```python
from build123d import *

# Parameters (mm, degrees)
SKETCH_1_R          = 1.1
SKETCH_1_R_2        = 1.35
EXTRUDE_1_DEPTH     = 3
SKETCH_2_R          = 1.6
CUT_EXTRUDE_1_DEPTH = 177.943493805
CUT_EXTRUDE_2_DEPTH = 177.943493805
FILLET_1_R          = 3
FILLET_2_R          = 1
FILLET_3_R          = 20


with BuildPart() as part:
    # 草图1 → 凸台-拉伸1 (new body)
    with BuildSketch(Plane(origin=(0, 0, 0), x_dir=(1, 0, 0), z_dir=(0, 1, 0))):
        Polygon((20, 120), (20, 80), (110, 80), (110, 120), (130, 120), (130, 0), (0, 0), (0, 120), align=None)
        with Locations(Location((10, 115, 0), (0, 0, 270))):
            Circle(SKETCH_1_R, mode=Mode.SUBTRACT)
        with Locations(Location((120, 115, 0), (0, 0, 90))):
            Circle(SKETCH_1_R, mode=Mode.SUBTRACT)
        with Locations(Location((10, 100, 0), (0, 0, 270))):
            Circle(SKETCH_1_R, mode=Mode.SUBTRACT)
        with Locations(Location((120, 100, 0), (0, 0, 90))):
            Circle(SKETCH_1_R, mode=Mode.SUBTRACT)
        with Locations(Location((10, 85, 0), (0, 0, 270))):
            Circle(SKETCH_1_R, mode=Mode.SUBTRACT)
        with Locations(Location((120, 85, 0), (0, 0, 90))):
            Circle(SKETCH_1_R, mode=Mode.SUBTRACT)
        with Locations(Location((10, 70, 0), (0, 0, 270))):
            Circle(SKETCH_1_R, mode=Mode.SUBTRACT)
        with Locations(Location((120, 70, 0), (0, 0, 90))):
            Circle(SKETCH_1_R, mode=Mode.SUBTRACT)
        with Locations(Location((10, 55, 0), (0, 0, 270))):
            Circle(SKETCH_1_R, mode=Mode.SUBTRACT)
        with Locations(Location((120, 55, 0), (0, 0, 90))):
            Circle(SKETCH_1_R, mode=Mode.SUBTRACT)
        with Locations(Location((10, 40, 0), (0, 0, 270))):
            Circle(SKETCH_1_R, mode=Mode.SUBTRACT)
        with Locations(Location((120, 40, 0), (0, 0, 90))):
            Circle(SKETCH_1_R, mode=Mode.SUBTRACT)
        with Locations(Location((50, 57.5, 0), (0, 0, 270))):
            Circle(SKETCH_1_R_2, mode=Mode.SUBTRACT)
        with Locations(Location((50, 43.5, 0), (0, 0, 270))):
            Circle(SKETCH_1_R_2, mode=Mode.SUBTRACT)
        with Locations(Location((80, 43.5, 0), (0, 0, 90))):
            Circle(SKETCH_1_R_2, mode=Mode.SUBTRACT)
        with Locations(Location((80, 57.5, 0), (0, 0, 90))):
            Circle(SKETCH_1_R_2, mode=Mode.SUBTRACT)
    extrude(amount=EXTRUDE_1_DEPTH)

    # 草图2 → 切除-拉伸1 (cut, through all)
    with BuildSketch(Plane.XZ):
        with Locations(Location((24, -7.85, 0), (0, 0, 270))):
            Circle(SKETCH_2_R)
        with Locations(Location((35, -7.85, 0), (0, 0, 90))):
            Circle(SKETCH_2_R)
        with Locations(Location((35, -67.85, 0), (0, 0, 270))):
            Circle(SKETCH_2_R)
        with Locations(Location((24, -67.85, 0), (0, 0, 90))):
            Circle(SKETCH_2_R)
        with Locations(Location((95, -67.85, 0), (0, 0, 90))):
            Circle(SKETCH_2_R)
        with Locations(Location((106, -67.85, 0), (0, 0, 270))):
            Circle(SKETCH_2_R)
        with Locations(Location((95, -7.85, 0), (0, 0, 270))):
            Circle(SKETCH_2_R)
        with Locations(Location((106, -7.85, 0), (0, 0, 90))):
            Circle(SKETCH_2_R)
        Polygon((37.954915028, -15.35), (29.5, -32.259830056), (21.045084972, -15.35), align=None)
        Polygon((19.5, -23.440169944), (26.704915028, -37.85), (19.5, -52.259830056), align=None)
        Polygon((29.5, -43.440169944), (21.045084972, -60.35), (37.954915028, -60.35), align=None)
        Polygon((90.5, -23.440169944), (97.704915028, -37.85), (90.5, -52.259830056), align=None)
        Polygon((39.5, -23.440169944), (39.5, -52.259830056), (32.295084972, -37.85), align=None)
        Polygon((100.5, -43.440169944), (92.045084972, -60.35), (108.954915028, -60.35), align=None)
        Polygon((110.5, -23.440169944), (103.295084972, -37.85), (110.5, -52.259830056), align=None)
        Polygon((92.045084972, -15.35), (108.954915028, -15.35), (100.5, -32.259830056), align=None)
        Polygon((54.545084972, -13.5), (75.454915028, -13.5), (65, -34.409830056), align=None)
        Polygon((53, -21.590169944), (62.204915028, -40), (53, -58.409830056), align=None)
        Polygon((65, -45.590169944), (76.079915028, -67.75), (53.920084972, -67.75), align=None)
        Polygon((77, -21.590169944), (77, -58.409830056), (67.795084972, -40), align=None)
    extrude(amount=-CUT_EXTRUDE_1_DEPTH, mode=Mode.SUBTRACT)

    # 草图3 → 切除-拉伸2 (cut, through all)
    with BuildSketch(Plane(origin=(0, 3, 0), x_dir=(1, 0, 0), z_dir=(0, 1, 0))):
        Polygon((17, 0), (0, 40), (0, 0), align=None)
        Polygon((113, 0), (130, 40), (130, 0), align=None)
    extrude(amount=-CUT_EXTRUDE_2_DEPTH, mode=Mode.SUBTRACT)

    # 圆角1
    fillet_1_edges = [part.edges().sort_by_distance(p)[0] for p in [
        (0, 1.5, -120),
        (20, 1.5, -120),
        (110, 1.5, -120),
        (130, 1.5, -120),
        (17, 1.5, 0),
        (0, 1.5, -40),
        (113, 1.5, 0),
        (130, 1.5, -40),
    ]]
    fillet(fillet_1_edges, radius=FILLET_1_R)

    # 圆角2
    fillet_2_edges = [part.edges().sort_by_distance(p)[0] for p in [
        (90.5, 1.5, -52.259830056),
        (90.5, 1.5, -23.440169944),
        (97.704915028, 1.5, -37.85),
        (19.5, 1.5, -52.259830056),
        (19.5, 1.5, -23.440169944),
        (26.704915028, 1.5, -37.85),
        (21.045084972, 1.5, -15.35),
        (37.954915028, 1.5, -15.35),
        (29.5, 1.5, -32.259830056),
        (39.5, 1.5, -52.259830056),
        (32.295084972, 1.5, -37.85),
        (39.5, 1.5, -23.440169944),
        (53.920084972, 1.5, -67.75),
        (65, 1.5, -45.590169944),
        (76.079915028, 1.5, -67.75),
        (100.5, 1.5, -32.259830056),
        (92.045084972, 1.5, -15.35),
        (108.954915028, 1.5, -15.35),
        (100.5, 1.5, -43.440169944),
        (108.954915028, 1.5, -60.35),
        (92.045084972, 1.5, -60.35),
        (110.5, 1.5, -23.440169944),
        (110.5, 1.5, -52.259830056),
        (103.295084972, 1.5, -37.85),
        (37.954915028, 1.5, -60.35),
        (21.045084972, 1.5, -60.35),
        (29.5, 1.5, -43.440169944),
        (65, 1.5, -34.409830056),
        (54.545084972, 1.5, -13.5),
        (75.454915028, 1.5, -13.5),
        (77, 1.5, -58.409830056),
        (67.795084972, 1.5, -40),
        (77, 1.5, -21.590169944),
        (53, 1.5, -58.409830056),
        (53, 1.5, -21.590169944),
        (62.204915028, 1.5, -40),
    ]]
    fillet(fillet_2_edges, radius=FILLET_2_R)

    # 圆角3
    fillet_3_edges = [part.edges().sort_by_distance(p)[0] for p in [
        (20, 1.5, -80),
        (110, 1.5, -80),
    ]]
    fillet(fillet_3_edges, radius=FILLET_3_R)


solid = part.part
```
Input: part model. Units: mm. Frame: model coordinates. A direction names the side the tool comes from. Coordinates: 2 decimals unless noted, no trailing zeros. Write each loop counter-clockwise with the first axis right and the second up, starting at its lowest first coordinate (ties: lowest second). Pieces come first, ordered by that corner, then holes. Notation, with made-up numbers: (19.5, 46) -> (49.5, 46) arc R36 cw to (49.5, 82) -> close; hole circle Ø4 at (13, 6.25). An arc over 180 degrees is marked (long way). Write each question's results on one line, items separated by ' | '.
Item 1: Mould query, pull axis Z, two halves, no side actions, for faces 4 (the flat face through (8.343, 1.521, -20.369)), 5 (the flat face through (104.86, 1.48, -52.16)), 6 (the flat face through (51, 3, -61)). Classes: +Z half, -Z half, draft (parallel to the pull), parting line (faces both ways), or undercut.
Conclusion:
face 4: +Z half | face 5: undercut | face 6: draft
Item 2: Section query D-D on y = 1.35. Count the separate pieces of the cut face and the enclosed holes in it, plus the area to 3 significant figures.
Conclusion:
separate pieces: 1 | enclosed holes: 36 | area: 9,610 mm^2
Item 3: Material intervals for probe 1 along X at (y, z) = (1.05, -67.85); probe 2 along Z at (x, y) = (31.5, 0.85); probe 3 along Z at (x, y) = (24.5, 2.6), sorted ascending.
Conclusion:
probe 1: x = 0 to 22.4, 25.6 to 33.4, 36.6 to 93.4, 96.6 to 104.4, 107.6 to 130 | probe 2: z = -81.9 to -60.35, -47.44 to -28.26, -15.35 to 0 | probe 3: z = -87.36 to -69.37, -66.33 to -60.35, -53.44 to -42.26, -33.44 to -22.26, -15.35 to -9.37, -6.33 to 0
Item 4: Pin query (flat end, axial travel): pin 1 Ø0.9 at (x, y) = (31, 1) entering from -Z; pin 2 Ø12 at (x, z) = (109, -96) entering from -Y. Return the tip coordinate at first contact, or that it passes through.
Conclusion:
pin 1: stops at z = -82.37 | pin 2: stops at y = 0
Item 5: Section query A-A on z = -109.5. Return loops of the section in (x, y), plus the area to 3 significant figures.
Conclusion:
outline: (0, 0) -> (20, 0) -> (20, 3) -> (0, 3) -> close; (110, 0) -> (130, 0) -> (130, 3) -> (110, 3) -> close | area: 120 mm^2
Item 6: Set-up query: faces 1 (the flat face through (94.9, 1.48, -32.24)), 2 (the flat face through (66, 1, 0)), 3 (the flat face through (20, 1, -109)). Return all of +Z, -Z, +X, -X, +Y, -Y with unobstructed straight access to the full face (end or side cutting, diameter ignored); none if empty.
Conclusion:
face 1: +Y, -Y | face 2: +Z, +X, -X, +Y, -Y | face 3: -Z, +Y, -Y
Item 7: Section query C-C on z = -21.5. Return loops of the section in (x, y).
Conclusion:
outline: (7.86, 0) -> (24.12, 0) -> (24.12, 3) -> (7.86, 3) -> close; (34.88, 0) -> (58.55, 0) -> (58.55, 3) -> (34.88, 3) -> close; (71.45, 0) -> (95.12, 0) -> (95.12, 3) -> (71.45, 3) -> close; (105.88, 0) -> (122.14, 0) -> (122.14, 3) -> (105.88, 3) -> close
Item 8: Section query B-B on z = -7.85. Return loops of the section in (x, y).
Conclusion:
outline: (13.66, 0) -> (22.4, 0) -> (22.4, 3) -> (13.66, 3) -> close; (25.6, 0) -> (33.4, 0) -> (33.4, 3) -> (25.6, 3) -> close; (36.6, 0) -> (93.4, 0) -> (93.4, 3) -> (36.6, 3) -> close; (96.6, 0) -> (104.4, 0) -> (104.4, 3) -> (96.6, 3) -> close; (107.6, 0) -> (116.34, 0) -> (116.34, 3) -> (107.6, 3) -> close
